from build123d import *

# Parameters (mm, degrees)
SKETCH1_W           = 120
SKETCH1_H           = 120
BOSS_EXTRUDE1_DEPTH = 8
CUT_EXTRUDE1_REACH  = 87.229
SKETCH2_R           = 30.5
CHAMFER1_SIZE       = 2
CUT_EXTRUDE2_REACH  = 87.229
SKETCH3_R           = 5
CHAMFER2_SIZE       = 5
M5_TAPPED_HOLE1_D   = 4.2


with BuildPart() as part:
    # Sketch1 → Boss-Extrude1 (new body)
    with BuildSketch(Plane(origin=(0, 0, 0), x_dir=(1, 0, 0), z_dir=(0, 1, 0))):
        Rectangle(SKETCH1_W, SKETCH1_H)
    extrude(amount=BOSS_EXTRUDE1_DEPTH)

    # Sketch2 → Cut-Extrude1 (cut, up to next)
    with BuildSketch(Plane(origin=(0, 8, 0), x_dir=(1, 0, 0), z_dir=(0, 1, 0)), mode=Mode.PRIVATE) as cut_extrude1_sk1:
        with Locations(Location((0, 0, 0), (0, 0, 270))):
            Circle(SKETCH2_R)
    cut_extrude1_tool1 = extrude(cut_extrude1_sk1.sketch, amount=-CUT_EXTRUDE1_REACH, mode=Mode.PRIVATE) & part.part
    add(cut_extrude1_tool1.solids().sort_by_distance((0, 8, 0))[0], mode=Mode.SUBTRACT)

    # Chamfer1
    chamfer1_edges = [part.edges().sort_by_distance(p)[0] for p in [
        (0, 8, -30.5),
    ]]
    chamfer(chamfer1_edges, length=CHAMFER1_SIZE)

    # Sketch3 → Cut-Extrude2 (cut, up to next)
    with BuildSketch(Plane(origin=(0, 8, 0), x_dir=(1, 0, 0), z_dir=(0, 1, 0)), mode=Mode.PRIVATE) as cut_extrude2_sk1:
        with Locations(Location((-50, 50, 0), (0, 0, 270))):
            Circle(SKETCH3_R)
    cut_extrude2_tool1 = extrude(cut_extrude2_sk1.sketch, amount=-CUT_EXTRUDE2_REACH, mode=Mode.PRIVATE) & part.part
    # Sketch3 → Cut-Extrude2 (cut, up to next)
    with BuildSketch(Plane(origin=(0, 8, 0), x_dir=(1, 0, 0), z_dir=(0, 1, 0)), mode=Mode.PRIVATE) as cut_extrude2_sk2:
        with Locations(Location((50, 50, 0), (0, 0, 270))):
            Circle(SKETCH3_R)
    cut_extrude2_tool2 = extrude(cut_extrude2_sk2.sketch, amount=-CUT_EXTRUDE2_REACH, mode=Mode.PRIVATE) & part.part
    # Sketch3 → Cut-Extrude2 (cut, up to next)
    with BuildSketch(Plane(origin=(0, 8, 0), x_dir=(1, 0, 0), z_dir=(0, 1, 0)), mode=Mode.PRIVATE) as cut_extrude2_sk3:
        with Locations(Location((-50, -50, 0), (0, 0, 270))):
            Circle(SKETCH3_R)
    cut_extrude2_tool3 = extrude(cut_extrude2_sk3.sketch, amount=-CUT_EXTRUDE2_REACH, mode=Mode.PRIVATE) & part.part
    # Sketch3 → Cut-Extrude2 (cut, up to next)
    with BuildSketch(Plane(origin=(0, 8, 0), x_dir=(1, 0, 0), z_dir=(0, 1, 0)), mode=Mode.PRIVATE) as cut_extrude2_sk4:
        with Locations(Location((50, -50, 0), (0, 0, 270))):
            Circle(SKETCH3_R)
    cut_extrude2_tool4 = extrude(cut_extrude2_sk4.sketch, amount=-CUT_EXTRUDE2_REACH, mode=Mode.PRIVATE) & part.part
    add(cut_extrude2_tool1.solids().sort_by_distance((-50, 8, -50))[0], mode=Mode.SUBTRACT)
    add(cut_extrude2_tool2.solids().sort_by_distance((50, 8, -50))[0], mode=Mode.SUBTRACT)
    add(cut_extrude2_tool3.solids().sort_by_distance((-50, 8, 50))[0], mode=Mode.SUBTRACT)
    add(cut_extrude2_tool4.solids().sort_by_distance((50, 8, 50))[0], mode=Mode.SUBTRACT)

    # Chamfer2
    chamfer2_edges = [part.edges().sort_by_distance(p)[0] for p in [
        (-60, 4, -60),
        (60, 4, -60),
        (60, 4, 60),
        (-60, 4, 60),
    ]]
    chamfer(chamfer2_edges, length=CHAMFER2_SIZE)

    # M5 Tapped Hole1 (through all)
    with Locations(Plane(origin=(0, 8, 0), x_dir=(1, 0, 0), z_dir=(0, 1, 0))):
        with Locations((-35.5, 0), (35.5, 0)):
            Hole(M5_TAPPED_HOLE1_D / 2)


solid = part.part
Read the model definition and answer for the solid it produces. Units are mm, in the model's axes. Coordinates: 2 decimals unless noted, no trailing zeros. Loops run counter-clockwise (first coordinate to the right, second up) from the corner with the lowest first, then second, coordinate; pieces in that order, holes last. Notation, with made-up numbers: (75, 86.5) - (95, 86.5) arc R24 ccw to (95, 101.5) - close; hole circle Ø11 at (76.5, 78.5). An arc over 180 degrees is marked (long way). Answer in a Markdown table with one row per item.
Q1. Find section A-A on z = 50. Write down the section's boundary in (x, y).
Here are the results:
| item | result |
|---|---|
| outline | (-60, 0) - (-55, 0) - (-55, 8) - (-60, 8) - close; (-45, 0) - (45, 0) - (45, 8) - (-45, 8) - close; (55, 0) - (60, 0) - (60, 8) - (55, 8) - close |
Q2. Find section B-B on x = 50. Write down the section's boundary in (y, z), plus the area to 3 significant figures.
Here are the results:
| item | result |
|---|---|
| outline | (0, -60) - (8, -60) - (8, -55) - (0, -55) - close; (0, -45) - (8, -45) - (8, 45) - (0, 45) - close; (0, 55) - (8, 55) - (8, 60) - (0, 60) - close |
| area | 800 mm^2 |
Q3. Find section C-C on z = 0. Write down the section's boundary in (x, y).
Here are the results:
| item | result |
|---|---|
| outline | (-60, 0) - (-37.6, 0) - (-37.6, 8) - (-60, 8) - close; (-33.4, 0) - (-30.5, 0) - (-30.5, 6) - (-32.5, 8) - (-33.4, 8) - close; (30.5, 0) - (33.4, 0) - (33.4, 8) - (32.5, 8) - (30.5, 6) - close; (37.6, 0) - (60, 0) - (60, 8) - (37.6, 8) - close |
Q4. Given P1, Ø9, axis at x = -50, z = -50, coming from the +Y side, flat-ended and moving along its own axis, determine where the tip first touches the part or whether it passes through.
Here are the results:
| item | result |
|---|---|
| P1 | passes through |
Q5. Find section D-D on x = -35.5. Write down the section's boundary in (y, z), plus the area to 3 significant figures.
Here are the results:
| item | result |
|---|---|
| outline | (0, -60) - (8, -60) - (8, -2.1) - (0, -2.1) - close; (0, 2.1) - (8, 2.1) - (8, 60) - (0, 60) - close |
| area | 926 mm^2 |
Q6. The mould has two halves that part along X. Classify faces 1 (the cylindrical face through (-33.4, 3.94, -0.09)), 2 (the flat face through (58, 4, 57)), 3 (the flat face through (-57, 4, 58)), 4 (the flat face through (-14, 0, -28)): pulls with the +X half, pulls with the -X half, needs draft (parallel to the pull), parting line crosses it, or undercut.
Here are the results:
| item | result |
|---|---|
| face 1 | undercut |
| face 2 | pulls with the +X half |
| face 3 | pulls with the -X half |
| face 4 | needs draft |
Q7. Straight lines are drawn through the part: line 1 along X through (y, z) = (5, -50); line 2 along X through (y, z) = (5.75, 48.5); line 3 along X through (y, z) = (6, -15). For each, find the intervals that lie inside material, in ascending order. Write a range as [from, to].
Here are the results:
| item | result |
|---|---|
| line 1 | x = [-60, -55], [-45, 45], [55, 60] |
| line 2 | x = [-60, -54.77], [-45.23, 45.23], [54.77, 60] |
| line 3 | x = [-60, -26.56], [26.56, 60] |
